Can you work these out from the drawing? Everything is in mm from the part's minimum corner. Round coordinates to 2 decimals unless told otherwise and drop trailing zeros. Loops run counter-clockwise (first coordinate to the right, second up) from the corner with the lowest first, then second, coordinate; pieces in that order, holes last. Notation, with made-up numbers: (-35, 1) -> (-17, 1) arc R19 ccw to (-17, 12) -> close; hole circle Ø6 at (84.5, 64.5). An arc over 180 degrees is marked (long way). One line per item, written item: value.
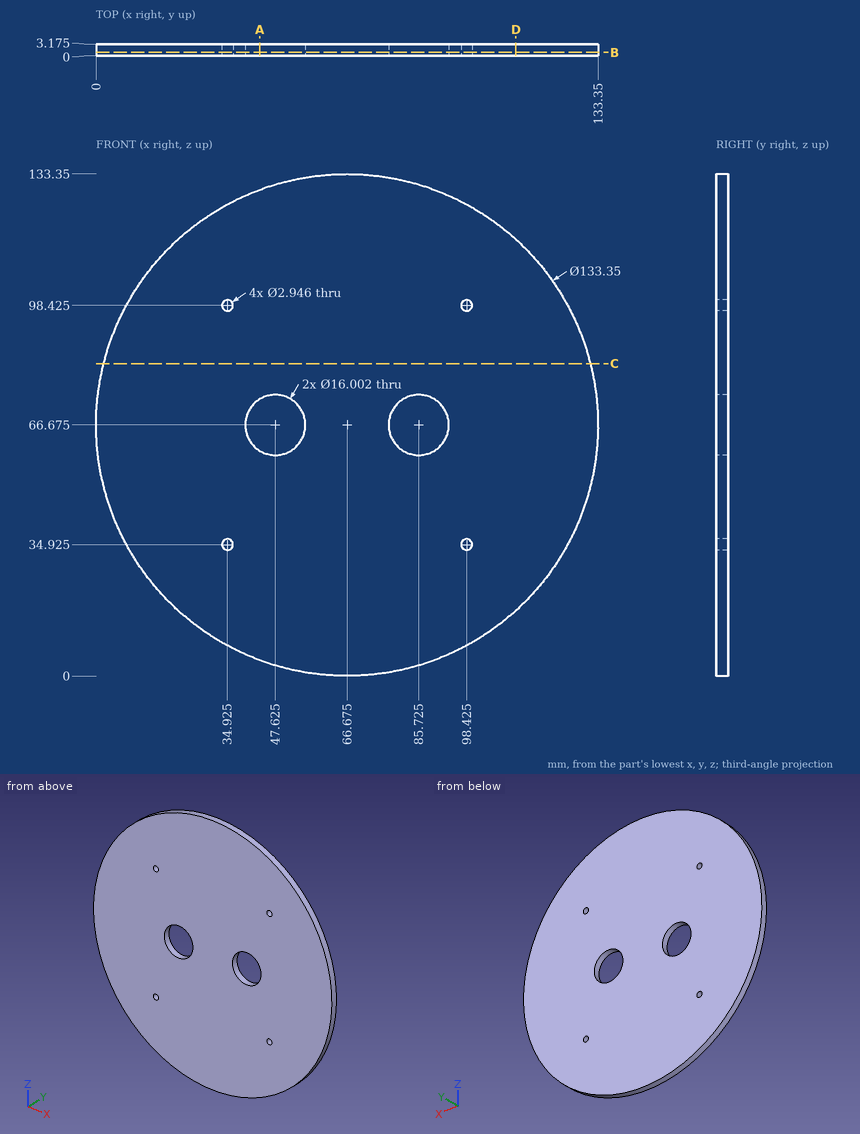
(1) Imagine slicing it at D-D on x = 111.5. Write out the boundary of the cut face in (y, z) (1 decimal).
Results below:
outline: (0, 17.3) -> (3.2, 17.3) -> (3.2, 116) -> (0, 116) -> close
(2) Imagine slicing it at A-A on x = 43.5. Write out the boundary of the cut face in (y, z) (1 decimal).
Results below:
outline: (0, 4.2) -> (3.2, 4.2) -> (3.2, 59.8) -> (0, 59.8) -> close; (0, 73.5) -> (3.2, 73.5) -> (3.2, 129.2) -> (0, 129.2) -> close
(3) For pin 1 Ø1.5 at (y, z) = (2.5, 19) entering from -X; pin 2 Ø1.5 at (x, y) = (60.5, 2) entering from +Z; pin 3 Ø1.5 at (y, z) = (0.5, 88) entering from +X, each with a flat end and sliding along its axis, tell me the tip position at first contact or that it passes through.
Results below:
pin 1: stops at x = 19.31
pin 2: stops at z = 133.13
pin 3: stops at x = 130.1
(4) Please list where these lines run through material, in increasing order: L1, parallel to Z at x = 99, y = 1.3; L2, parallel to X at y = 1.7, z = 62 (1 decimal); L3, parallel to Z at x = 99.5, y = 0.2.
Results below:
L1: z = 8.36 to 33.57, 36.28 to 97.07, 99.78 to 124.99
L2: x = 0.2 to 41.1, 54.1 to 79.2, 92.2 to 133.2
L3: z = 8.64 to 33.92, 35.93 to 97.42, 99.43 to 124.71
(5) Imagine slicing it at C-C on z = 83. Write out the boundary of the cut face in (x, y) (1 decimal).
Results below:
outline: (2, 0) -> (131.3, 0) -> (131.3, 3.2) -> (2, 3.2) -> close
(6) Imagine slicing it at B-B on y = 0.95. Give the number of separate pieces and of enclosed holes in the cut face, then the cut area to 3 significant figures.
Results below:
separate pieces: 1
enclosed holes: 6
area: 13,500 mm²
